from build123d import *

# Parameters (mm, degrees)
SKETCH_1_R      = 25
EXTRUDE_1_DEPTH = 500
FILLET_1_R      = 25
SKETCH_3_R      = 20
EXTRUDE_2_DEPTH = 100


with BuildPart() as part:
    # 草图1 → 凸台-拉伸1 (new body)
    with BuildSketch(Plane(origin=(0, 0, 0), x_dir=(1, 0, 0), z_dir=(0, 1, 0))):
        with Locations(Location((0, 0, 0), (0, 0, 270))):
            Circle(SKETCH_1_R)
    extrude(amount=EXTRUDE_1_DEPTH)

    # 圆角1
    fillet_1_edges = [part.edges().sort_by_distance(p)[0] for p in [
        (0, 500, -25),
    ]]
    fillet(fillet_1_edges, radius=FILLET_1_R)

    # 草图3 → 凸台-拉伸2 (add)
    with BuildSketch(Plane.XY):
        with Locations(Location((0, 465, 0), (0, 0, 149.999999999))):
            Circle(SKETCH_3_R)
    extrude(amount=EXTRUDE_2_DEPTH)


solid = part.part
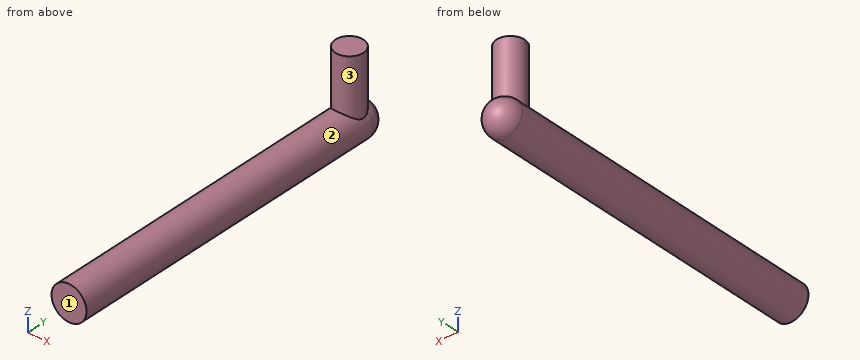
Can you work these out from the model? Positions are in its coordinate system, mm. Face numbers are marked on the shaded views. A direction names the side the tool comes from. Give positions to 0.01 mm unless a question says otherwise; leave off trailing zeros. Loops run counter-clockwise (first coordinate to the right, second up) from the corner with the lowest first, then second, coordinate; pieces in that order, holes last. Notation, with made-up numbers: (19, 67.25) - (70, 67.25) arc R34 ccw to (70, 101.25) - close; hole circle Ø9 at (-28, 48). An arc over 180 degrees is marked (long way). Return JSON: item names as keys, results as strings.
1. I want a section at A-A on x = 0. Please give me the cut outline in (y, z).
Output values:
{"outline": "(0, -25) - (475, -25) arc R25 ccw to (485, 22.91) - (485, 100) - (445, 100) - (445, 25) - (0, 25) - close"}
2. I want a section at B-B on y = 465. Please give me the cut outline in (x, z), and give its area (3 significant figures).
Output values:
{"outline": "(-20, 15) arc R25 ccw (long way) to (20, 15) - (20, 100) - (-20, 100) - close", "area": "5,080 mm²"}
3. If I drill on line 1 (Y direction, x = -1, z = -1); line 2 (Y direction, x = 2, z = 94); line 3 (Z direction, x = 5.5, y = 359), over which ranges is the centre line in solid material (lowest first)?
Output values:
{"line 1": "y = 0 to 499.96", "line 2": "y = 445.1 to 484.9", "line 3": "z = -24.39 to 24.39"}
4. I'm going to push flat-ended pins straight in: pin 1 Ø2 at (x, y) = (-9, 274) entering from -Z; pin 2 Ø6 at (x, y) = (13, 148.5) entering from +Z; pin 3 Ø6 at (x, y) = (11.5, 221) entering from +Z. Where does each tip first touch, or does it pass through?
Output values:
{"pin 1": "stops at z = -23.69", "pin 2": "stops at z = 22.91", "pin 3": "stops at z = 23.51"}
5. For the marked faces 1, 2 and 3, which set-ups out of +Z, -Z, +X, -X, +Y, -Y let a thin tool reach every point of the face, with its end or its side?
Output values:
{"face 1": "+Z, -Z, +X, -X, -Y", "face 2": "-Y", "face 3": "+Z"}
6. I want a section at C-C on z = 49.5. Please give me the cut outline in (x, y).
Output values:
{"outline": "circle Ø40 at (0, 465)"}
